Part model, mm, in its own coordinate system. Face numbers are marked on the shaded views. A direction names the side the tool comes from. Coordinates: 2 decimals unless noted, no trailing zeros. Loops run counter-clockwise (first coordinate to the right, second up) from the corner with the lowest first, then second, coordinate; pieces in that order, holes last. Notation, with made-up numbers: (50.25, 78) -> (70.25, 78) arc R19 cw to (70.25, 90) -> close; hole circle Ø11 at (4, 14.25). An arc over 180 degrees is marked (long way). Use one line per item in the form item = value. Start each with the question number.
(1) Drill centre lines: L1, parallel to X at y = -11.2, z = 12.5; L2, parallel to X at y = 0, z = 8.75; L3, parallel to Z at x = 0, y = -11.4. Where is each one in solid material? Low to high. Write a range as [from, to].
(2) Band-saw the part on A-A on x = 0. Give the cut face in (y, z), then the cut area to 3 significant figures.
(3) Pin check, flat tips, straight feed: P1, Ø8, axis at x = 7.5, y = 9.5, coming from the -Z side; P2, Ø11, axis at x = 0, z = 12.5, coming from the -Y side; P3, Ø4.5, axis at x = -1, y = 1, coming from the -Z side. Stop position of each tip, or through.
(4) Mould opens along X. For the marked faces 3, 4 and 5 say: +X half, -X half, draft (parallel to the pull), parting line (faces both ways), or undercut.
(5) Band-saw the part on C-C on y = -3.75. Give the cut face in (x, z).
(6) 3-axis set-ups, long thin cutter, end or side, ignore diameter. For the marked faces 1 and 2: which of +Z, -Z, +X, -X, +Y, -Y reach the whole face in a straight line?
Autodesk Inventor part; units mm, degrees
ref_plane "YZ Plane" through (0, 0, 0) normal (1, 0, 0) x (0, 1, 0)
ref_plane "XZ Plane" through (0, 0, 0) normal (0, 1, 0) x (-1, 0, 0)
ref_plane "XY Plane" through (0, 0, 0) normal (0, 0, 1) x (1, 0, 0)
sketch "Sketch2" plane through (0, 0, 0) normal (0, 0, 1) x (1, 0, 0)
  circle A0 centre (0, 0) radius 7.5
  line L0 (12.5, 12.5) -> (-12.5, 12.5)
  line L1 (-12.5, 12.5) -> (-12.5, -12.5)
  line L2 (-12.5, -12.5) -> (12.5, -12.5)
  line L3 (12.5, -12.5) -> (12.5, 12.5)
  line L4 (7.5, 7.5) -> (-7.5, 7.5)
  line L5 (-7.5, 7.5) -> (-7.5, -7.5)
  line L6 (-7.5, -7.5) -> (7.5, -7.5)
  line L7 (7.5, -7.5) -> (7.5, 7.5)
  dimension "d0" = 15
  dimension "d1" = 25
  dimension "d2" = 25
  dimension "d3" = 12.5
  dimension "d4" = 12.5
  dimension "d5" = 15
  dimension "d6" = 15
extrude "Extrusion1" add sketch "Sketch2" along normal blind 25
sketch "Sketch3" plane through (-7.5, -7.5, 0) normal (0, 1, 0) x (1, 0, 0)
  line L0 (15, 0) -> (15, -25)
  line L1 (0, 0) -> (0, -25)
  line L2 (15, -20) -> (0, -20)
  line L3 (0, -20) -> (0, -5)
  line L4 (0, -5) -> (15, -5)
  line L5 (15, -5) -> (15, -20)
  circle A0 centre (7.5, -12.5) radius 6
  point P0 (7.5, 0)
  dimension "d9" = 15
  dimension "d10" = 12
extrude "Extrusion2" cut sketch "Sketch3" against normal blind 5 contours A0
chamfer "Chamfer1" distance 1.5 angle 45 1 edges at (-6, -7.5, 12.5)
sketch "Sketch4" plane through (0, 0, 25) normal (0, 0, 1) x (1, 0, 0)
  line L0 (-12.5, 12.5) -> (-12.5, -12.5)
  line L1 (-12.5, -12.5) -> (12.5, -12.5)
  line L2 (-12.5, 12.5) -> (12.5, 12.5)
  line L3 (12.5, 12.5) -> (12.5, -12.5)
  line L4 (12.5, -12.5) -> (-12.5, -12.5)
  line L5 (-12.5, -12.5) -> (-12.5, 12.5)
  point P0 (0, 0)
extrude "Extrusion3" add sketch "Sketch4" along normal blind 5
properties part number "Example Slider"
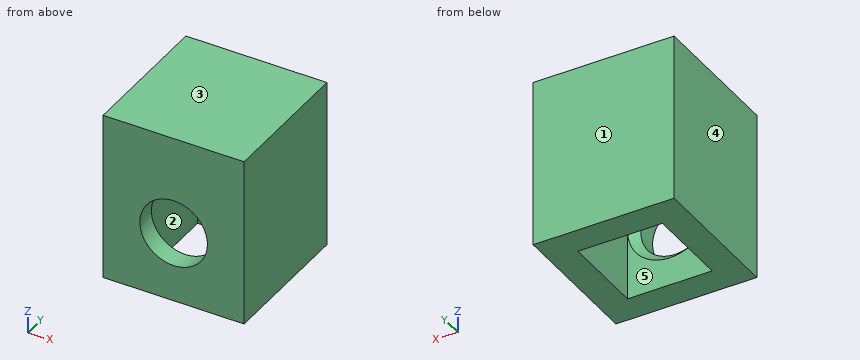
A:
q1.L1 = [-12.5, -6], [6, 12.5]
q1.L2 = [-12.5, -7.5], [7.5, 12.5]
q1.L3 = [0, 6.5], [18.5, 30]
q2.outline = (-12.5, 0) -> (-7.5, 0) -> (-7.5, 5) -> (-9, 6.5) -> (-12.5, 6.5) -> close; (-12.5, 18.5) -> (-9, 18.5) -> (-7.5, 20) -> (-7.5, 25) -> (7.5, 25) -> (7.5, 0) -> (12.5, 0) -> (12.5, 30) -> (-12.5, 30) -> close
q2.area = 313 mm²
q3.P1 = 0
q3.P2 = 7.5
q3.P3 = 25
q4.face_3 = draft
q4.face_4 = -X half
q4.face_5 = undercut
q5.outline = (-12.5, 0) -> (-7.5, 0) -> (-7.5, 25) -> (7.5, 25) -> (7.5, 0) -> (12.5, 0) -> (12.5, 30) -> (-12.5, 30) -> close
q6.face_1 = +Z, -Z, +X, -X, +Y
q6.face_2 = -Z
